Could you check a few things on this model? Use its own coordinates, in mm. A direction names the side the tool comes from. Coordinates: 2 decimals unless noted, no trailing zeros. Loops run counter-clockwise (first coordinate to the right, second up) from the corner with the lowest first, then second, coordinate; pieces in that order, holes last.
Autodesk Inventor part; units mm, degrees
ref_plane "YZ Plane" through (0, 0, 0) normal (1, 0, 0) x (0, 1, 0)
ref_plane "XZ Plane" through (0, 0, 0) normal (0, 1, 0) x (-1, 0, 0)
ref_plane "XY Plane" through (0, 0, 0) normal (0, 0, 1) x (1, 0, 0)
sketch "Szkic7" plane through (0, 0, 0) normal (0, 0, 1) x (1, 0, 0)
  circle A0 centre (0, 0) radius 13.2205
  dimension "d35" = 26.441
extrude "Wyciągnięcie proste2" add sketch "Szkic7" along normal mid plane 19.175
chamfer "Faza2" distance 1 angle 45 1 edges at (-13.2205, 0, 9.5875)
sketch "Szkic9" plane through (0, 0, 9.5875) normal (0, 0, 1) x (1, 0, 0)
  circle A0 centre (0, 0) radius 12.2205
extrude "Wyciągnięcie proste3" add sketch "Szkic9" along normal blind 1.625
sketch "Szkic10" plane through (0, 0, 11.2125) normal (0, 0, 1) x (1, 0, 0)
  line L0 (-8.6603, 15) -> (8.6603, 15)
  line L1 (8.6603, 15) -> (17.3205, 0)
  line L2 (17.3205, 0) -> (8.6603, -15)
  line L3 (8.6603, -15) -> (-8.6603, -15)
  line L4 (-8.6603, -15) -> (-17.3205, 0)
  line L5 (-17.3205, 0) -> (-8.6603, 15)
  line L6 (0, 18.5087) -> (0, -18.5087) construction
  line L7 (-18.5087, 0) -> (18.5087, 0) construction
  point P0 (0, 0)
  point P1 (0, 0)
  point P2 (0, 15)
  dimension "d44" = 30
extrude "Wyciągnięcie proste4" add sketch "Szkic10" along normal blind 5.2
sketch "Szkic12" plane through (0, 0, 0) normal (0, 1, 0) x (-1, 0, 0)
  line L0 (0, -2.1463) -> (0, 12.8775) construction
  line L1 (-8.6603, 11.2125) -> (-8.6603, 16.4125) construction
  line L2 (-17.3205, 16.4125) -> (-8.6603, 16.4125) construction
  line L3 (-17.3205, 11.2125) -> (-17.3205, 16.4125)
  line L4 (-17.3205, 15.8766) -> (-15.3205, 16.4125)
  line L5 (-17.3205, 16.4125) -> (-8.6603, 16.4125)
  line L6 (-17.3205, 11.2125) -> (-8.6603, 11.2125)
  point P0 (0, 0)
  dimension "d50" = 15
  dimension "d51" = 2
revolve "Obrót2" cut sketch "Szkic12" angle 360 about axis through (0, 0, -10) along (0, 0, 1)
thread "Gwint3"
chamfer "Faza3" distance 1 angle 45 1 edges at (-13.2205, 0, -9.5875)
equation "\"d35\" = OD"
equation "\"d36\" = 0.7375 * L"
equation "\"d42\" = 0.0625 * L"
equation "\"d44\" = SW"
equation "\"d45\" = 0.2 * L"
equation "\"d51\" = 0.0666667 * SW"
equation "\"SzerokośćGięciaPodcięcia\" = Grubość"
equation "\"RozmiarPodcięciaNarożnika\" = 4 * Grubość"
equation "\"PromieńPrzejścia\" = PromieńGięcia"
equation "\"Rozmiar_promienia_Jacobiego\" = PromieńGięcia"
equation "\"Wielk_odstępu\" = Grubość"
equation "\"d2\" = PromieńGięcia"
equation "\"d23\" = PromieńGięcia"
equation "\"OD\" = 26.441"
equation "\"SW\" = 30"
equation "\"L\" = 26"
properties part number "Korek sześciokątny BSP 3/4'' L=26" material "304"
1) Imagine slicing it at B-B on z = 4.5. List the corners of the cut face in (x, y) for me.
2) Imagine slicing it at A-A on x = 0. List the corners of the cut face in (y, z) for me.
3) Will these pins go through, and if not, where does the flat tip stop? pin 1 (6 mm diameter, centred on y = -11.5, z = 11, fed in from -X); pin 2 (10 mm diameter, centred on x = 13, z = 6.5, fed in from +Y); pin 3 (1.5 mm diameter, centred on y = -9, z = 12, fed in from -X).
4) For faces 5 (the flat face through (-13.051, 7.395, 13.776)), 6 (the flat face through (9, -9, 11.212)), which set-ups out of +Z, -Z, +X, -X, +Y, -Y let a thin tool reach every point of the face, with its end or its side?
5) If I drill on L1, parallel to Z at x = -4, y = -13; L2, parallel to Y at x = 0.5, z = -6.5; L3, parallel to Z at x = 5.5, y = 11.5, over which ranges is the centre line in solid material (lowest first)?
6) Imagine slicing it at C-C on z = 10.5. List the corners of the cut face in (x, y) for me, plus the area to 3 significant figures.
7) We'd pull the mould along Z, two halves only. Please class faces 1 (the flat face through (0, 0, -9.588)), 2 (the conical face through (-15.89, -0.07, 16.26)), 3 (the cylindrical face through (-1.591, -12.117, 10.389)), 4 (the cylindrical face through (6.1, -11.73, 0.12)): released by +Z, released by -Z, zero draft, split by the parting line, or undercut.
Solved:
1. outline: circle Ø26.44 at (0, 0)
2. outline: (-15, 11.21) - (-12.22, 11.21) - (-12.22, 9.59) - (-13.22, 8.59) - (-13.22, -8.59) - (-12.22, -9.59) - (12.22, -9.59) - (13.22, -8.59) - (13.22, 8.59) - (12.22, 9.59) - (12.22, 11.21) - (15, 11.21) - (15, 16.41) - (-15, 16.41) - close
3. pin 1: stops at x = -12.41
3. pin 2: stops at y = 10.53
3. pin 3: stops at x = -12.56
4. face 5: +Z, -Z, -X, +Y
4. face 6: none
5. L1: z = 11.21 to 16.41
5. L2: y = -13.21 to 13.21
5. L3: z = -9.06 to 9.06, 11.21 to 16.41
6. outline: circle Ø24.44 at (0, 0)
6. area: 469 mm2
7. face 1: released by -Z
7. face 2: released by +Z
7. face 3: undercut
7. face 4: zero draft
